Autodesk Inventor part; units mm, degrees
ref_plane "YZ Plane" through (0, 0, 0) normal (1, 0, 0) x (0, 1, 0)
ref_plane "XZ Plane" through (0, 0, 0) normal (0, 1, 0) x (-1, 0, 0)
ref_plane "XY Plane" through (0, 0, 0) normal (0, 0, 1) x (1, 0, 0)
sketch "スケッチ1" plane through (0, 0, 0) normal (0, 0, 1) x (1, 0, 0)
  line L0 (7.5, 15) -> (-7.5, 15)
  line L1 (-7.5, 15) -> (-7.5, -15)
  line L2 (-7.5, -15) -> (7.5, -15)
  line L3 (7.5, -15) -> (7.5, 15)
  line L4 (7.5, 15) -> (-7.5, -15) construction
  line L5 (-7.5, 15) -> (7.5, -15) construction
  line L6 (-5.5, 13) -> (5.5, 13)
  line L7 (5.5, 13) -> (5.5, -13)
  line L8 (5.5, -13) -> (-5.5, -13)
  line L9 (-5.5, -13) -> (-5.5, 13)
  point P0 (0, 0)
  dimension "d0" = 15
  dimension "d1" = 30
  dimension "d2" = 2
extrude "押し出し1" add sketch "スケッチ1" along normal blind 1132
sketch "スケッチ2" plane through (-7.5, 15, 1132) normal (0, 1, 0) x (1, 0, 0)
  circle A0 centre (7.5, 1122) radius 1.6
  circle A1 centre (7.5, 1112) radius 1.6
  line L0 (15, 1132) -> (0, 1132)
  circle A2 centre (7.5, 7.5) radius 1.6
  circle A3 centre (7.5, 22.5) radius 1.6
  line L1 (15, 0) -> (0, 0)
  point P0 (7.5, 1132)
  point P1 (7.5, 1132)
  point P2 (7.5, 0)
  dimension "d5" = 3.2
  dimension "d6" = 3.2
  dimension "d7" = 10
  dimension "d8" = 10
  dimension "d9" = 3.2
  dimension "d10" = 3.2
  dimension "d11" = 15
  dimension "d12" = 7.5
extrude "押し出し2" cut sketch "スケッチ2" against normal through all
properties part number "上昇機構_角柱1" material "アルミニウム 6061"
For this review, take the finished solid that the model builds, in its own axes (mm). Coordinates: 2 decimals unless noted, no trailing zeros. Order: outer loops, then holes, each group sorted by start corner. A loop starts at its lowest first (then second) coordinate and runs counter-clockwise, first axis right, second up. Notation, with made-up numbers: (-3, 45.25) -> (3, 45.25) arc R20 ccw to (3, 59.25) -> close; hole circle Ø5 at (2.25, 28). An arc over 180 degrees is marked (long way). Answer as CSV lines item,"result".
Q1. We need section A-A (y = -4.25). State the section outline as (x, z) points, plus the area to 3 significant figures.
Model answer:
outline,"(-7.5, 0) -> (-5.5, 0) -> (-5.5, 1132) -> (-7.5, 1132) -> close; (5.5, 0) -> (7.5, 0) -> (7.5, 1132) -> (5.5, 1132) -> close"
area,"4,530 mm2"
Q2. Wall thickness on line 1 along Z through (x, y) = (0, -13.95); line 2 along Y through (x, z) = (-4, 824); line 3 along X through (y, z) = (-5.75, 268.5): over which ranges is each line inside the solid? List them lowest first. Write a range as [from, to].
Model answer:
line 1,"z = [0, 8.4], [11.6, 18.4], [21.6, 1107.9], [1111.1, 1122.9], [1126.1, 1132]"
line 2,"y = [-15, -13], [13, 15]"
line 3,"x = [-7.5, -5.5], [5.5, 7.5]"
Q3. We need section B-B (z = 761). State the section outline as (x, y) points, plus the area to 3 significant figures.
Model answer:
outline,"(-7.5, -15) -> (7.5, -15) -> (7.5, 15) -> (-7.5, 15) -> close; hole (-5.5, -13) -> (5.5, -13) -> (5.5, 13) -> (-5.5, 13) -> close"
area,"164 mm2"
Q4. Draft analysis for pull direction X (two halves, no side actions). For faces 1 (the face through (5.5, 0, 558)), 2 (the face through (7.5, 0, 558)), 3 (the face through (-7.5, 0, 558)), state which applies: released by +X, released by -X, zero draft, split by the parting line, or undercut.
Model answer:
face 1,"undercut"
face 2,"released by +X"
face 3,"released by -X"
Q5. Clearance check with a flat-ended pin moving along its axis: pin 1 Ø3 at (x, z) = (0, 1109.5) entering from +Y. State where the tip first meets the part, or that it passes through.
Model answer:
pin 1,"passes through"
